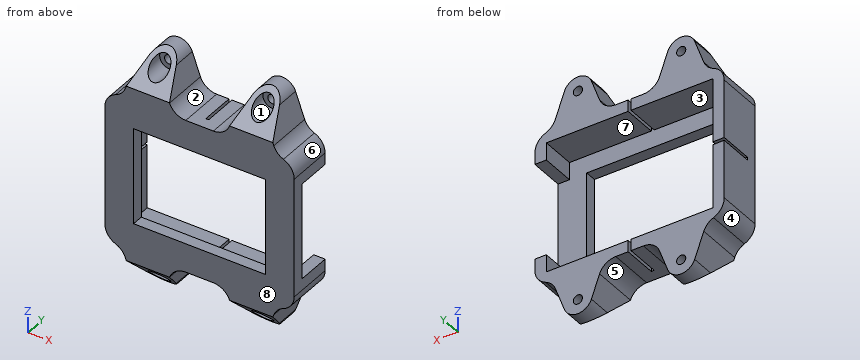
```python
from build123d import *

# Parameters (mm, degrees)
SKETCH_1_W            = 66
SKETCH_1_H            = 53.5
SKETCH_1_W_2          = 58
SKETCH_1_H_2          = 45.5
SKETCH_1_W_3          = 46
SKETCH_1_H_3          = 33.5
EXTRUDE_1_DEPTH       = 4
EXTRUDE_START         = 4
SKETCH_1_4_W          = 66
SKETCH_1_4_H          = 53.5
SKETCH_1_4_W_2        = 58
SKETCH_1_4_H_2        = 45.5
EXTRUDE_2_DEPTH       = 12
SKETCH_2_R            = 1.6
EXTRUDE_3_DEPTH       = 5
CHAMFER_1_OUTLINE_R   = 1.6
CHAMFER_1_DEPTH       = 11
CHAMFER_START         = -14
CHAMFER_1_2_OUTLINE_W = 54
CHAMFER_1_2_OUTLINE_H = 60.830212793
CHAMFER_1_2_DEPTH     = 8.343145751
CHAMFER_START_2       = 35.001785669
CHAMFER_1_3_OUTLINE_W = 54
CHAMFER_1_3_OUTLINE_H = 8.169787207
CHAMFER_1_3_DEPTH     = 18.384776311
SKETCH_4_R            = 3.3
CUT_EXTRUDE_1_DEPTH   = 11
SKETCH_5_W            = 1
SKETCH_5_H            = 4
SKETCH_5_W_2          = 4
SKETCH_5_H_2          = 1
CUT_EXTRUDE_1_2_DEPTH = 12
FILLET_1_R            = 6
FILLET_2_R            = 6
SKETCH_6_W            = 33.396299262
SKETCH_6_H            = 12
CUT_EXTRUDE_2_DEPTH   = 8


with BuildPart() as part:
    # 草图1 → 凸台-拉伸1 (new body)
    # profile 1 of 2: a face of its own
    with BuildSketch(Plane(origin=(0, 0, 0), x_dir=(1, 0, 0), z_dir=(0, 1, 0))):
        with Locations((0, 22.75)):
            Rectangle(SKETCH_1_W, SKETCH_1_H)
        with Locations((0, 22.75)):
            Rectangle(SKETCH_1_W_2, SKETCH_1_H_2, mode=Mode.SUBTRACT)
    # profile 2 of 2: a face of its own
    with BuildSketch(Plane(origin=(0, 0, 0), x_dir=(1, 0, 0), z_dir=(0, 1, 0))):
        with Locations((0, 22.75)):
            Rectangle(SKETCH_1_W_2, SKETCH_1_H_2)
        with Locations((0, 22.75)):
            Rectangle(SKETCH_1_W_3, SKETCH_1_H_3, mode=Mode.SUBTRACT)
    extrude(amount=EXTRUDE_1_DEPTH)

    # 草图1<4> → 凸台-拉伸2 (add)
    with BuildSketch(Plane(origin=(0, 0, 0), x_dir=(1, 0, 0), z_dir=(0, 1, 0)).offset(EXTRUDE_START)):
        with Locations((0, 22.75)):
            Rectangle(SKETCH_1_4_W, SKETCH_1_4_H)
        with Locations((0, 22.75)):
            Rectangle(SKETCH_1_4_W_2, SKETCH_1_4_H_2, mode=Mode.SUBTRACT)
    extrude(amount=EXTRUDE_2_DEPTH)

    # 草图2 → 凸台-拉伸3 (add)
    # profile 1 of 4: a face of its own
    with BuildSketch(Plane(origin=(0, 16, 0), x_dir=(1, 0, 0), z_dir=(0, 1, 0))):
        with BuildLine():
            Line((13.30663094, 61.224032154), (9, 49.5))
            Line((9, 49.5), (27, 49.5))
            Line((27, 49.5), (22.69336906, 61.224032154))
            ThreePointArc((22.69336906, 61.224032154), (18, 64.5), (13.30663094, 61.224032154))
        make_face()
        with Locations(Location((18, 59.5, 0), (0, 0, 270))):
            Circle(SKETCH_2_R, mode=Mode.SUBTRACT)
    # profile 2 of 4: a face of its own
    with BuildSketch(Plane(origin=(0, 16, 0), x_dir=(1, 0, 0), z_dir=(0, 1, 0))):
        with BuildLine():
            Line((-27, 49.5), (-22.69336906, 61.224032154))
            ThreePointArc((-22.69336906, 61.224032154), (-18, 64.5), (-13.30663094, 61.224032154))
            Line((-13.30663094, 61.224032154), (-9, 49.5))
            Line((-9, 49.5), (-27, 49.5))
        make_face()
        with Locations(Location((-18, 59.5, 0), (0, 0, 90))):
            Circle(SKETCH_2_R, mode=Mode.SUBTRACT)
    # profile 3 of 4: a face of its own
    with BuildSketch(Plane(origin=(0, 16, 0), x_dir=(1, 0, 0), z_dir=(0, 1, 0))):
        with BuildLine():
            Line((-13.30663094, -15.724032154), (-9, -4))
            Line((-9, -4), (-27, -4))
            Line((-27, -4), (-22.69336906, -15.724032154))
            ThreePointArc((-22.69336906, -15.724032154), (-18, -19), (-13.30663094, -15.724032154))
        make_face()
        with Locations(Location((-18, -14, 0), (0, 0, 270))):
            Circle(SKETCH_2_R, mode=Mode.SUBTRACT)
    # profile 4 of 4: a face of its own
    with BuildSketch(Plane(origin=(0, 16, 0), x_dir=(1, 0, 0), z_dir=(0, 1, 0))):
        with BuildLine():
            Line((27, -4), (22.69336906, -15.724032154))
            ThreePointArc((22.69336906, -15.724032154), (18, -19), (13.30663094, -15.724032154))
            Line((13.30663094, -15.724032154), (9, -4))
            Line((9, -4), (27, -4))
        make_face()
        with Locations(Location((18, -14, 0), (0, 0, 90))):
            Circle(SKETCH_2_R, mode=Mode.SUBTRACT)
    extrude(amount=-EXTRUDE_3_DEPTH)

    # 倒角1: read off the stored shape, not the designer's step
    # 倒角1 outline → 倒角1 (add)
    # profile 1 of 4: a face of its own
    with BuildSketch(Plane(origin=(0, 0, 0), x_dir=(1, 0, 0), z_dir=(0, 1, 0))):
        with BuildLine():
            Line((9, 49.5), (27, 49.5))
            Line((27, 49.5), (22.69336906, 61.224032154))
            ThreePointArc((22.69336906, 61.224032154), (18, 64.5), (13.30663094, 61.224032154))
            Line((13.30663094, 61.224032154), (9, 49.5))
        make_face()
        with Locations((18, 59.5)):
            Circle(CHAMFER_1_OUTLINE_R, mode=Mode.SUBTRACT)
    # profile 2 of 4: a face of its own
    with BuildSketch(Plane(origin=(0, 0, 0), x_dir=(1, 0, 0), z_dir=(0, 1, 0))):
        with BuildLine():
            Line((-27, 49.5), (-9, 49.5))
            Line((-9, 49.5), (-13.30663094, 61.224032154))
            ThreePointArc((-13.30663094, 61.224032154), (-18, 64.5), (-22.69336906, 61.224032154))
            Line((-22.69336906, 61.224032154), (-27, 49.5))
        make_face()
        with Locations((-18, 59.5)):
            Circle(CHAMFER_1_OUTLINE_R, mode=Mode.SUBTRACT)
    # profile 3 of 4: a face of its own
    with BuildSketch(Plane(origin=(0, 0, 0), x_dir=(1, 0, 0), z_dir=(0, 1, 0))):
        with BuildLine():
            Line((-27, -4), (-22.69336906, -15.724032154))
            ThreePointArc((-22.69336906, -15.724032154), (-18, -19), (-13.30663094, -15.724032154))
            Line((-13.30663094, -15.724032154), (-9, -4))
            Line((-9, -4), (-27, -4))
        make_face()
        with Locations((-18, -14)):
            Circle(CHAMFER_1_OUTLINE_R, mode=Mode.SUBTRACT)
    # profile 4 of 4: a face of its own
    with BuildSketch(Plane(origin=(0, 0, 0), x_dir=(1, 0, 0), z_dir=(0, 1, 0))):
        with BuildLine():
            Line((27, -4), (9, -4))
            Line((9, -4), (13.30663094, -15.724032154))
            ThreePointArc((13.30663094, -15.724032154), (18, -19), (22.69336906, -15.724032154))
            Line((22.69336906, -15.724032154), (27, -4))
        make_face()
        with Locations((18, -14)):
            Circle(CHAMFER_1_OUTLINE_R, mode=Mode.SUBTRACT)
    extrude(amount=CHAMFER_1_DEPTH)

    # Chamfer 1 2 outline → Chamfer 1 2 (cut)
    with BuildSketch(Plane(origin=(0, 0, 0), x_dir=(1, 0, 0), z_dir=(0, 0.707106781186544, -0.707106781186551)).offset(CHAMFER_START)):
        with Locations((0, 7.415106397)):
            Rectangle(CHAMFER_1_2_OUTLINE_W, CHAMFER_1_2_OUTLINE_H)
    extrude(amount=CHAMFER_1_2_DEPTH, mode=Mode.SUBTRACT)

    # Chamfer 1 3 outline → Chamfer 1 3 (cut)
    with BuildSketch(Plane(origin=(0, 0, 0), x_dir=(1, 0, 0), z_dir=(0, 0.707106781186544, -0.707106781186551)).offset(CHAMFER_START_2)):
        with Locations((0, 41.915106397)):
            Rectangle(CHAMFER_1_3_OUTLINE_W, CHAMFER_1_3_OUTLINE_H)
    extrude(amount=CHAMFER_1_3_DEPTH, mode=Mode.SUBTRACT)

    # 草图4 → Cut-Extrude 1 (cut)
    with BuildSketch(Plane.XZ):
        with Locations(Location((-18, 14, 0), (0, 0, 270))):
            Circle(SKETCH_4_R)
        with Locations(Location((18, 14, 0), (0, 0, 270))):
            Circle(SKETCH_4_R)
        with Locations(Location((18, -59.5, 0), (0, 0, 270))):
            Circle(SKETCH_4_R)
        with Locations(Location((-18, -59.5, 0), (0, 0, 270))):
            Circle(SKETCH_4_R)
    extrude(amount=-CUT_EXTRUDE_1_DEPTH, mode=Mode.SUBTRACT)

    # 草图5 → Cut-Extrude 1 2 (cut)
    with BuildSketch(Plane(origin=(0, 16, 0), x_dir=(1, 0, 0), z_dir=(0, 1, 0))):
        with Locations((0, 47.5)):
            Rectangle(SKETCH_5_W, SKETCH_5_H)
        with Locations((31, 22.75)):
            Rectangle(SKETCH_5_W_2, SKETCH_5_H_2)
        with Locations((0, -2)):
            Rectangle(SKETCH_5_W, SKETCH_5_H)
        with Locations((-31, 22.75)):
            Rectangle(SKETCH_5_W_2, SKETCH_5_H_2)
    extrude(amount=-CUT_EXTRUDE_1_2_DEPTH, mode=Mode.SUBTRACT)

    # 圆角1
    fillet_1_edges = [part.edges().sort_by_distance(p)[0] for p in [
        (-33, 8, -49.5),
        (-33, 8, 4),
        (33, 8, -49.5),
        (33, 8, 4),
    ]]
    fillet(fillet_1_edges, radius=FILLET_1_R - 0.0001)  # a hair under: the kernel refuses the full size

    # 圆角2
    fillet_2_edges = [part.edges().sort_by_distance(p)[0] for p in [
        (27, 5.5, -49.5),
        (9, 5.5, -49.5),
        (-9, 5.5, -49.5),
        (-27, 5.5, -49.5),
        (-27, 5.5, 4),
        (-9, 5.5, 4),
        (9, 5.5, 4),
        (27, 5.5, 4),
    ]]
    fillet(fillet_2_edges, radius=FILLET_2_R)

    # 草图6 → 切除-拉伸2 (cut)
    with BuildSketch(Plane(origin=(33, 0, 0), x_dir=(0, 0, -1), z_dir=(1, 0, 0))):
        with Locations((22.75, 10)):
            Rectangle(SKETCH_6_W, SKETCH_6_H)
    extrude(amount=-CUT_EXTRUDE_2_DEPTH, mode=Mode.SUBTRACT)


solid = part.part
```
Work out the finished part from the listing and answer in its coordinate system (mm). Face numbers are marked on the shaded views. A direction names the side the tool comes from. Give positions to 0.01 mm unless a question says otherwise; leave off trailing zeros. Loops run counter-clockwise (first coordinate to the right, second up) from the corner with the lowest first, then second, coordinate; pieces in that order, holes last. Notation, with made-up numbers: (65.5, 35.25) -> (84.5, 35.25) arc R11 ccw to (84.5, 44.25) -> close; hole circle Ø7 at (0.5, 78.5). An arc over 180 degrees is marked (long way). Write item = value, one per line. Start each with the question number.
(1) Find section C-C on z = -59.5. Give the vertices of the cut face in (x, y).
(2) Which of the six approach directions +Z, -Z, +X, -X, +Y, -Y give full straight-line access (tool end or side, diameter ignored) to the marked faces 1, 2, 3 and 4?
(3) The mould has two halves that part along Z. Classify the marked faces 5, 6, 7 and 8: +Z half, -Z half, draft (parallel to the pull), parting line (faces both ways), or undercut.
(4) Find section D-D on y = 5.75. Give the number of separate pieces and of enclosed holes in the cut face, and give its area (3 significant figures).
(5) Find section B-B on x = -9.5. Give the vertices of the cut face in (y, z), and give its area (3 significant figures).
(6) Find the intervals of material crossed by probe 1 along Z at (x, y) = (-18, 5); probe 2 along Z at (x, y) = (16, 10.5); probe 3 along X at (y, z) = (14.2, 14), in increasing order. Write a range as from..to.
(7) Find section A-A on z = -33. Give the vertices of the cut face in (x, y).
(8) Given pin 1 Ø1 at (x, y) = (-9.5, 11.5) entering from -Z; pin 2 Ø6 at (x, y) = (25, 5.5) entering from -Z; pin 3 Ø2 at (x, y) = (31.5, 13) entering from +Z, each flat-ended and moving along its own axis, determine where each tip first touches the part or whether it passes through.
From the geometry:
q1.outline = (-23.33, 6) -> (-21.3, 6) -> (-21.3, 11) -> (-19.6, 11) -> (-19.6, 16) -> (-23.33, 16) -> close; (-16.4, 11) -> (-14.7, 11) -> (-14.7, 6) -> (-12.67, 6) -> (-12.67, 16) -> (-16.4, 16) -> close; (12.67, 6) -> (14.7, 6) -> (14.7, 11) -> (16.4, 11) -> (16.4, 16) -> (12.67, 16) -> close; (19.6, 11) -> (21.3, 11) -> (21.3, 6) -> (23.33, 6) -> (23.33, 16) -> (19.6, 16) -> close
q2.face_1 = -Y
q2.face_2 = +Z, +Y, -Y
q2.face_3 = +Y
q2.face_4 = -Z, -X, +Y, -Y
q3.face_5 = -Z half
q3.face_6 = +Z half
q3.face_7 = undercut
q3.face_8 = draft
q4.separate_pieces = 4
q4.enclosed_holes = 0
q4.area = 1,230 mm^2
q5.outline = (0, -51.76) -> (16, -51.76) -> (16, -45.5) -> (4, -45.5) -> (4, -39.5) -> (0, -39.5) -> close; (0, -6) -> (4, -6) -> (4, 0) -> (16, 0) -> (16, 6.26) -> (0, 6.26) -> close
q5.area = 248 mm^2
q6.probe_1 = -56.2..-45.5, 0..10.7
q6.probe_2 = -64..-62.12, -56.88..-45.5, 0..11.38, 16.62..18.5
q6.probe_3 = -23.33..-19.6, -16.4..-12.67, 12.67..16.4, 19.6..23.33
q7.outline = (-33, 0) -> (-23, 0) -> (-23, 4) -> (-29, 4) -> (-29, 16) -> (-33, 16) -> close; (23, 0) -> (33, 0) -> (33, 4) -> (23, 4) -> close
q8.pin_1 = -52.49
q8.pin_2 = -61.01
q8.pin_3 = 2.87
